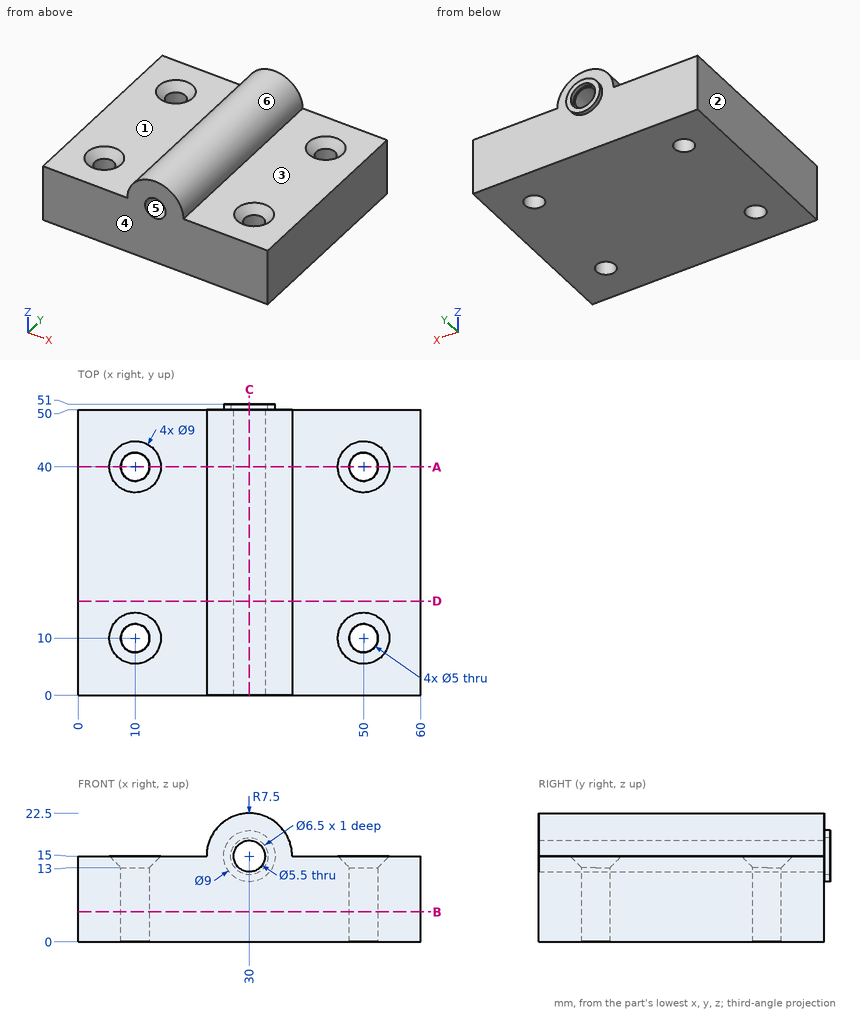
Geometry check sheet. Reference: drawing and pictorial views, mm from the part's lowest x, y, z. A direction names the side the tool comes from. Give positions to 0.01 mm unless a question says otherwise; leave off trailing zeros. Order: outer loops, then holes, each group sorted by start corner. A loop starts at its lowest first (then second) coordinate and runs counter-clockwise, first axis right, second up.
1. Access from +Z, -Z, +X, -X, +Y, -Y to the whole of each face (thin tool, end or side, straight path). Record for the marked faces 1, 2 and 3.
2. Thickness scan on L1, parallel to Y at x = 50, z = 9.75; L2, parallel to X at y = 10, z = 9; L3, parallel to Z at x = 30, y = 50.75. Record the ranges inside material, lowest first.
3. Section check B-B, the plane z = 5.25. Enter the section's corners in (x, y).
4. Release check for a two-part mould opening along Z. For the marked faces 4, 5 and 6 record: pulls with the +Z half, pulls with the -Z half, needs draft (parallel to the pull), parting line crosses it, or undercut.
5. Gauge pin test, flat ends, axial feed: pin 1 Ø12 at (x, y) = (39, 17) entering from +Z; pin 2 Ø1.5 at (x, y) = (47, 31) entering from +Z; pin 3 Ø1.5 at (x, z) = (42, 5.5) entering from +Y. Record the tip position at first contact, or that the pin passes through.
6. Section check C-C, the plane x = 30. Enter the section's corners in (y, z), and give its area (4 significant figures).
7. Section check A-A, the plane y = 40. Enter the section's corners in (x, z).
8. Section check D-D, the plane y = 16.5. Enter the section's corners in (x, z).
Values follow:
1. face 1: +Z, -X, +Y, -Y
1. face 2: +Z, -Z, -X, +Y, -Y
1. face 3: +Z, +X, +Y, -Y
2. L1: y = 0 to 7.5, 12.5 to 37.5, 42.5 to 50
2. L2: x = 0 to 7.5, 12.5 to 47.5, 52.5 to 60
2. L3: z = 10.5 to 11.75, 18.25 to 19.5
3. outline: (0, 0) - (60, 0) - (60, 50) - (0, 50) - close; hole circle Ø5 at (10, 10); hole circle Ø5 at (10, 40); hole circle Ø5 at (50, 10); hole circle Ø5 at (50, 40)
4. face 4: needs draft
4. face 5: undercut
4. face 6: pulls with the +Z half
5. pin 1: stops at z = 21.87
5. pin 2: stops at z = 15
5. pin 3: stops at y = 50
6. outline: (0, 0) - (50, 0) - (50, 10.5) - (51, 10.5) - (51, 11.75) - (50, 11.75) - (50, 12.25) - (0, 12.25) - close; (0, 17.75) - (50, 17.75) - (50, 18.25) - (51, 18.25) - (51, 19.5) - (50, 19.5) - (50, 22.5) - (0, 22.5) - close
6. area: 852.5 mm2
7. outline: (0, 0) - (7.5, 0) - (7.5, 13) - (5.5, 15) - (0, 15) - close; (12.5, 0) - (47.5, 0) - (47.5, 13) - (45.5, 15) - (37.5, 15) arc R7.5 ccw to (22.5, 15) - (14.5, 15) - (12.5, 13) - close; (52.5, 0) - (60, 0) - (60, 15) - (54.5, 15) - (52.5, 13) - close; hole circle Ø5.5 at (30, 15)
8. outline: (0, 0) - (60, 0) - (60, 15) - (37.5, 15) arc R7.5 ccw to (22.5, 15) - (0, 15) - close; hole circle Ø5.5 at (30, 15)
